The model under review builds one solid part; all positions refer to its coordinate system, in mm. Coordinates: 2 decimals unless noted, no trailing zeros. Write each loop counter-clockwise with the first axis right and the second up, starting at its lowest first coordinate (ties: lowest second). Pieces come first, ordered by that corner, then holes. Notation, with made-up numbers: (42, 16) - (94, 16) arc R19 ccw to (94, 42) - close; hole circle Ø4 at (1, -22). An arc over 180 degrees is marked (long way). Put each result on its own line as item: value.
from build123d import *

# Parameters (mm, degrees)
SKETCH_1_W      = 52
SKETCH_1_H      = 14
EXTRUDE_1_DEPTH = 2
FILLET_2_R      = 1


with BuildPart() as part:
    # 草图1 → 凸台-拉伸1 (new body)
    with BuildSketch(Plane.XY):
        with Locations((26, 7)):
            Rectangle(SKETCH_1_W, SKETCH_1_H)
    extrude(amount=EXTRUDE_1_DEPTH)

    # 圆角2
    fillet_2_edges = [part.edges().sort_by_distance(p)[0] for p in [
        (26, 0, 0),
        (0, 7, 0),
        (26, 14, 0),
        (52, 7, 0),
        (52, 0, 1),
        (0, 0, 1),
        (0, 14, 1),
        (52, 14, 1),
    ]]
    fillet(fillet_2_edges, radius=FILLET_2_R)

    # 草图6 → 切除-旋转4 (revolve, cut)
    with BuildSketch(Plane(origin=(26, 0, 0), x_dir=(0, 0, -1), z_dir=(1, 0, 0)), mode=Mode.PRIVATE) as cut_revolve_4_sk:
        Polygon((0, 10), (0, 11.4), (-1.1, 10.8), (-2, 10.8), (-2, 10), align=None)
    revolve(cut_revolve_4_sk.sketch.rotate(Axis((26, 10, 0), (0, 0, 1)), 90), axis=Axis((26, 10, 0), (0, 0, 1)), mode=Mode.SUBTRACT)

    # 草图5 → 切除-旋转5 (revolve, cut)
    with BuildSketch(Plane(origin=(26, 0, 0), x_dir=(0, 0, -1), z_dir=(1, 0, 0)), mode=Mode.PRIVATE) as cut_revolve_5_sk:
        Polygon((0, 4), (0, 2.6), (-1.1, 3.2), (-2, 3.2), (-2, 4), align=None)
    revolve(cut_revolve_5_sk.sketch.rotate(Axis((26, 4, 0), (0, 0, 1)), 180), axis=Axis((26, 4, 0), (0, 0, 1)), mode=Mode.SUBTRACT)


solid = part.part
1. The part is to be moulded in two halves that separate along X. For faces 1 (the cylindrical face through (0.285, 0.301, 1.507)), 2 (the flat face through (26, 7, 2)), 3 (the cylindrical face through (26, 3.2, 1.6)), 4 (the cylindrical face through (25.57, 9.325, 1.556)), say which applies: +X half, -X half, draft (parallel to the pull), parting line (faces both ways), or undercut.
Determined:
face 1: -X half
face 2: draft
face 3: undercut
face 4: undercut
2. Consider section D-D on x = 48.5. State the section outline as (y, z) points.
Determined:
outline: (0, 1) arc R1 ccw to (1, 0) - (13, 0) arc R1 ccw to (14, 1) - (14, 2) - (0, 2) - close
3. Consider section B-B on y = 4. State the section outline as (x, z) points, plus the area to 3 significant figures.
Determined:
outline: (0, 1) arc R1 ccw to (1, 0) - (24.6, 0) - (25.2, 1.1) - (25.2, 2) - (0, 2) - close; (26.8, 1.1) - (27.4, 0) - (51, 0) arc R1 ccw to (52, 1) - (52, 2) - (26.8, 2) - close
area: 99.7 mm^2
4. Consider section C-C on z = 0.35. State the section outline as (x, y) points.
Determined:
outline: (0.24, 1) arc R0.76 ccw to (1, 0.24) - (51, 0.24) arc R0.76 ccw to (51.76, 1) - (51.76, 13) arc R0.76 ccw to (51, 13.76) - (1, 13.76) arc R0.76 ccw to (0.24, 13) - close; hole circle Ø2.42 at (26, 4); hole circle Ø2.42 at (26, 10)
5. Consider section A-A on x = 26. State the section outline as (y, z) points.
Determined:
outline: (0, 1) arc R1 ccw to (1, 0) - (2.6, 0) - (3.2, 1.1) - (3.2, 2) - (0, 2) - close; (4.8, 1.1) - (5.4, 0) - (8.6, 0) - (9.2, 1.1) - (9.2, 2) - (4.8, 2) - close; (10.8, 1.1) - (11.4, 0) - (13, 0) arc R1 ccw to (14, 1) - (14, 2) - (10.8, 2) - close
6. To check wall thickness, follow probe 1 along Y at (x, z) = (26, 1.5); probe 2 along Y at (x, z) = (26, 0.6); probe 3 along X at (y, z) = (4, 1.45). State the ranges of each line that lie inside material, in increasing order.
Determined:
probe 1: y = 0 to 3.2, 4.8 to 9.2, 10.8 to 14
probe 2: y = 0.08 to 2.93, 5.07 to 8.93, 11.07 to 13.92
probe 3: x = 0 to 25.2, 26.8 to 52
